Could you check a few things on this drawing? It's one solid part, dimensions in mm from its lowest x, y, z. Coordinates: 2 decimals unless noted, no trailing zeros. Write each loop counter-clockwise with the first axis right and the second up, starting at its lowest first coordinate (ties: lowest second). Pieces come first, ordered by that corner, then holes. Notation, with made-up numbers: M 89,61.25 L 119,61.25 A11 cw 119,77.25 Z; hole C 7,-29.5 d6. An arc over 180 degrees is marked long. Use a Markdown table: item, result.
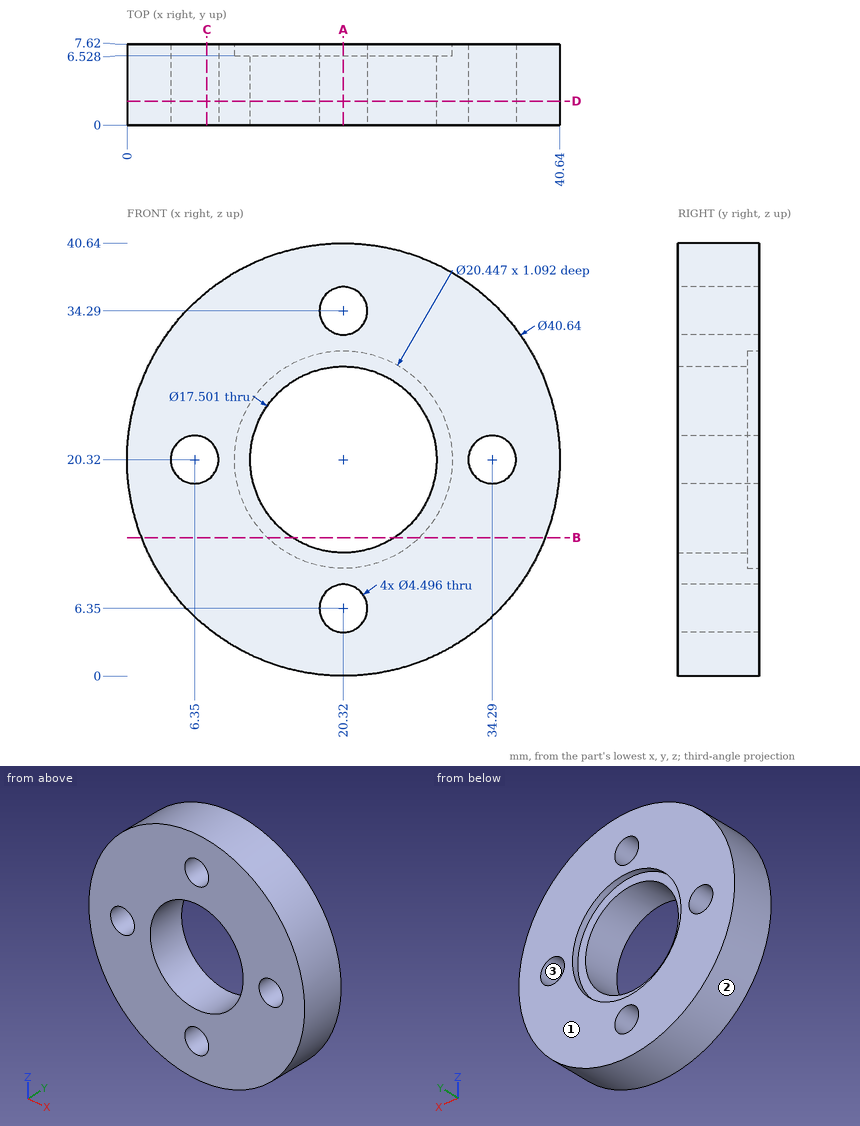
1. Suppose I cut it at B-B on z = 13. Write out the boundary of the cut face in (x, y) (1 decimal).
Answers follow:
| item | result |
|---|---|
| outline | M 1.4,0 L 15.5,0 L 15.5,6.5 L 13.2,6.5 L 13.2,7.6 L 1.4,7.6 Z; M 25.1,0 L 39.3,0 L 39.3,7.6 L 27.5,7.6 L 27.5,6.5 L 25.1,6.5 Z |
2. Suppose I cut it at A-A on x = 20.32. Write out the boundary of the cut face in (y, z).
Answers follow:
| item | result |
|---|---|
| outline | M 0,0 L 7.62,0 L 7.62,4.1 L 0,4.1 Z; M 0,8.6 L 7.62,8.6 L 7.62,10.1 L 6.53,10.1 L 6.53,11.57 L 0,11.57 Z; M 0,29.07 L 6.53,29.07 L 6.53,30.54 L 7.62,30.54 L 7.62,32.04 L 0,32.04 Z; M 0,36.54 L 7.62,36.54 L 7.62,40.64 L 0,40.64 Z |
3. I need wall thicknesses on probe 1 along Z at (x, y) = (20.32, 3.25); probe 2 along X at (y, z) = (2.25, 34.29) (1 decimal). Which ranges of each line are inside material? Lowest first, please.
Answers follow:
| item | result |
|---|---|
| probe 1 | z = 0 to 4.1, 8.6 to 11.57, 29.07 to 32.04, 36.54 to 40.64 |
| probe 2 | x = 5.6 to 18.1, 22.6 to 35.1 |
4. Suppose I cut it at D-D on y = 2.25. State how many separate pieces and enclosed holes the cut face has, and give its area (3 significant figures).
Answers follow:
| item | result |
|---|---|
| separate pieces | 1 |
| enclosed holes | 5 |
| area | 993 mm2 |
5. We'd pull the mould along Z, two halves only. Please class the marked faces 1, 2 and 3: +Z half, -Z half, draft (parallel to the pull), parting line (faces both ways), or undercut.
Answers follow:
| item | result |
|---|---|
| face 1 | draft |
| face 2 | parting line |
| face 3 | undercut |
6. Suppose I cut it at C-C on x = 7.5. Write out the boundary of the cut face in (y, z) (1 decimal).
Answers follow:
| item | result |
|---|---|
| outline | M 0,4.6 L 7.6,4.6 L 7.6,18.4 L 0,18.4 Z; M 0,22.3 L 7.6,22.3 L 7.6,36.1 L 0,36.1 Z |
7. Will these pins go through, and if not, where does the flat tip stop? pin 1 Ø6 at (x, z) = (16, 19.5) entering from +Y; pin 2 Ø4 at (x, y) = (28.5, 3) entering from +Z.
Answers follow:
| item | result |
|---|---|
| pin 1 | passes through |
| pin 2 | stops at z = 39.68 |
